from build123d import *

# Parameters (mm, degrees)
F0_R     = 20
F1_DEPTH = 125


with BuildPart() as f1:
    # F0 (on Top) → F1 (new body, symmetric)
    with BuildSketch(Plane.XY):
        Polygon((125, 95), (95, 125), (-95, 125), (-125, 95), (-125, 27.5), (-75, 27.5), (-75, -27.5), (-125, -27.5), (-125, -95), (-95, -125), (95, -125), (125, -95), align=None)
        with Locations((-75, -75)):
            Circle(F0_R, mode=Mode.SUBTRACT)
        with Locations((75, -75)):
            Circle(F0_R, mode=Mode.SUBTRACT)
        with Locations((-75, 75)):
            Circle(F0_R, mode=Mode.SUBTRACT)
        Polygon((-27.5, -75), (-27.5, 75), (27.5, 75), (27.5, 27.5), (75, 27.5), (75, -27.5), (27.5, -27.5), (27.5, -75), align=None, mode=Mode.SUBTRACT)
        with Locations((75, 75)):
            Circle(F0_R, mode=Mode.SUBTRACT)
    extrude(amount=F1_DEPTH, both=True)


solid = f1.part
Geometry check sheet. Reference: the model listing, model coordinates, mm. A direction names the side the tool comes from. Coordinates: 2 decimals unless noted, no trailing zeros. Order: outer loops, then holes, each group sorted by start corner. A loop starts at its lowest first (then second) coordinate and runs counter-clockwise, first axis right, second up. Notation, with made-up numbers: (54.25, -17) -> (108.25, -17) arc R27 ccw to (108.25, 5) -> close; hole circle Ø9 at (19.25, 56.5). An arc over 180 degrees is marked (long way). Use a Markdown table: item, result. Add a question column.
1. Mould release check, pull along Y, two halves, no side actions. Record for faces 1 (the face through (75, 0, 2)), 2 (the face through (110, 110, 2)), 3 (the face through (-30, 2, 125)): pulls with the +Y half, pulls with the -Y half, needs draft (parallel to the pull), parting line crosses it, or undercut.
2. Go/stop test with flat-tipped pins: pin 1 Ø24 at (x, y) = (75, 75) entering from -Z; pin 2 Ø4 at (y, z) = (-17, 54.5) entering from -X. Record where each tip stops, or that it passes through.
3. Cross-section at B-B (x = 63). Enter the section's corners in (y, z).
4. Material ranges on L1, parallel to X at y = 13, z = -86.5; L2, parallel to Y at x = -17, z = -103; L3, parallel to Y at x = 43, z = -78, recorded low to high.
5. Cross-section at A-A (y = 39). Enter the section's corners in (x, z), and give its area (4 significant figures).
6. Set-up check for faces 4 (the face through (-1, -125, 2)), 5 (the face through (-100, -27.5, 2)), 6 (the face through (0, 75, 2)): record each of +Z, -Z, +X, -X, +Y, -Y from which the full face is reachable in a straight line by a thin tool's end or side.
7. Cross-section at D-D (x = -20.5). Enter the section's corners in (y, z).
8. Cross-section at C-C (z = 29). Enter the section's corners in (x, y), and give its area (3 significant figures).
Filled sheet:
| question | item | result |
|---|---|---|
| 1 | face 1 | undercut |
| 1 | face 2 | pulls with the +Y half |
| 1 | face 3 | needs draft |
| 2 | pin 1 | through |
| 2 | pin 2 | x = -75 |
| 3 | outline | (-125, -125) -> (-91, -125) -> (-91, 125) -> (-125, 125) -> close; (-59, -125) -> (-27.5, -125) -> (-27.5, 125) -> (-59, 125) -> close; (27.5, -125) -> (59, -125) -> (59, 125) -> (27.5, 125) -> close; (91, -125) -> (125, -125) -> (125, 125) -> (91, 125) -> close |
| 4 | L1 | -75 to -27.5, 75 to 125 |
| 4 | L2 | -125 to -75, 75 to 125 |
| 4 | L3 | -125 to -27.5, 27.5 to 125 |
| 5 | outline | (-125, -125) -> (-27.5, -125) -> (-27.5, 125) -> (-125, 125) -> close; (27.5, -125) -> (125, -125) -> (125, 125) -> (27.5, 125) -> close |
| 5 | area | 48,750 mm2 |
| 6 | face 4 | +Z, -Z, +X, -X, -Y |
| 6 | face 5 | +Z, -Z, -X |
| 6 | face 6 | +Z, -Z |
| 7 | outline | (-125, -125) -> (-75, -125) -> (-75, 125) -> (-125, 125) -> close; (75, -125) -> (125, -125) -> (125, 125) -> (75, 125) -> close |
| 8 | outline | (-125, -95) -> (-95, -125) -> (95, -125) -> (125, -95) -> (125, 95) -> (95, 125) -> (-95, 125) -> (-125, 95) -> (-125, 27.5) -> (-75, 27.5) -> (-75, -27.5) -> (-125, -27.5) -> close; hole circle Ø40 at (-75, -75); hole circle Ø40 at (-75, 75); hole (-27.5, -75) -> (27.5, -75) -> (27.5, -27.5) -> (75, -27.5) -> (75, 27.5) -> (27.5, 27.5) -> (27.5, 75) -> (-27.5, 75) -> close; hole circle Ø40 at (75, -75); hole circle Ø40 at (75, 75) |
| 8 | area | 42,100 mm2 |
